The model under review builds one solid part; all positions refer to its coordinate system, in mm. A direction names the side the tool comes from. Coordinates: 2 decimals unless noted, no trailing zeros. Write each loop counter-clockwise with the first axis right and the second up, starting at its lowest first coordinate (ties: lowest second). Pieces come first, ordered by that corner, then holes. Notation, with made-up numbers: (14, 33) -> (72, 33) arc R14 cw to (72, 40) -> close; hole circle Ø9 at (8.5, -14.5). An arc over 180 degrees is marked (long way). Put each result on its own line as item: value. Start each with the question number.
from build123d import *

# Parameters (mm, degrees)
SKETCH_R          = 8.35
SKETCH_R_2        = 7.1
PAD_DEPTH         = 4
SKETCH001_W       = 35.5
SKETCH001_H       = 35.5
SKETCH001_R       = 6.6
PAD001_DEPTH      = 2
SKETCH002_W       = 4
SKETCH002_H       = 2
POCKET_DEPTH      = 25
POCKET_DEPTH_BACK = 25
FILLET002_R       = 0.5
SKETCH010_R       = 7.1
POCKET002_DEPTH   = 1


with BuildPart() as part:
    # Sketch → Pad (new body)
    with BuildSketch(Plane.XZ):
        Circle(SKETCH_R)
        Circle(SKETCH_R_2, mode=Mode.SUBTRACT)
    extrude(amount=PAD_DEPTH)

    # Sketch001 → Pad001 (join)
    with BuildSketch(Plane.XZ):
        with Locations((1.775, 0)):
            Rectangle(SKETCH001_W, SKETCH001_H)
        Circle(SKETCH001_R, mode=Mode.SUBTRACT)
    extrude(amount=-PAD001_DEPTH)

    # Sketch002 (on DatumPlane) → Pocket (cut, two sides)
    with BuildSketch(Plane.YZ) as pocket_sk:
        with Locations((-2, 0)):
            Rectangle(SKETCH002_W, SKETCH002_H)
    extrude(amount=-POCKET_DEPTH, mode=Mode.SUBTRACT)
    extrude(pocket_sk.sketch, amount=POCKET_DEPTH_BACK, mode=Mode.SUBTRACT)

    # Fillet002
    fillet002_edges = [part.edges().sort_by_distance(p)[0] for p in [
        (-15.975, 1, -17.75),
        (-15.975, 1, 17.75),
    ]]
    fillet(fillet002_edges, radius=FILLET002_R)

    # Sketch010 → Pocket002 (cut)
    with BuildSketch(Plane.XZ):
        Circle(SKETCH010_R)
    extrude(amount=-POCKET002_DEPTH, mode=Mode.SUBTRACT)


with BuildPart() as part_1:
    # Body placement: moved
    add(part.part.moved(Location((-2.5, -3, 0))))


solid = part_1.part
1. Tool access review of faces 1 (the cylindrical face through (4.272, -4.535, 2.133)), 2 (the flat face through (5, -5, 1)), 3 (the cylindrical face through (-2.67, -4.97, -8.35)): name each direction out of +Z, -Z, +X, -X, +Y, -Y from which nothing blocks a thin tool from reaching the whole face with its end or side.
2. Consider section D-D on z = -11. State the section outline as (x, y) points (3 decimals), then the cut area to 3 significant figures.
3. Consider section A-A on z = 0. State the section outline as (x, y) points (3 decimals), then the cut area to 3 significant figures.
4. Consider section B-B on x = -2.5. State the section outline as (y, z) points, then the cut area to 3 significant figures.
5. Wall thickness on line 1 (Z direction, x = -2.5, y = -4.5); line 2 (Z direction, x = -2.5, y = -1.5); line 3 (Y direction, x = -15, z = 12.5): over which ranges is each line inside the solid? List them lowest first. Write a range as from..to.
6. Insertion check: P1, Ø1.4, axis at x = 5.5, y = -6, coming from the -Z side; P2, Ø12, axis at x = -2.5, z = 0, coming from the -Y side; P3, Ø1, axis at x = 5.5, y = -4, coming from the +Z side; P4, Ø0.6, axis at x = -10.5, y = -5, coming from the +Z side. Each pin has a flat end and moves straight along its axis. Give the tip position at first contact, or say it passes through.
7. Consider section C-C on y = -4.8. State the section outline as (x, z) points, then the cut area to 3 significant figures.
Output values:
1. face 1: -Y
1. face 2: +X, -X, -Y
1. face 3: -Z, -Y
2. outline: (-18.475, -3) -> (17.025, -3) -> (17.025, -1) -> (-18.475, -1) -> close
2. area: 71.0 mm^2
3. outline: (-18.475, -3) -> (-9.6, -3) -> (-9.6, -2) -> (-9.1, -2) -> (-9.1, -1) -> (-18.475, -1) -> close; (4.1, -2) -> (4.6, -2) -> (4.6, -3) -> (17.025, -3) -> (17.025, -1) -> (4.1, -1) -> close
3. area: 43.6 mm^2
4. outline: (-7, -8.35) -> (-3, -8.35) -> (-3, -17.75) -> (-1, -17.75) -> (-1, -6.6) -> (-2, -6.6) -> (-2, -7.1) -> (-7, -7.1) -> close; (-7, 7.1) -> (-2, 7.1) -> (-2, 6.6) -> (-1, 6.6) -> (-1, 17.75) -> (-3, 17.75) -> (-3, 8.35) -> (-7, 8.35) -> close
4. area: 53.6 mm^2
5. line 1: z = -8.35..-7.1, 7.1..8.35
5. line 2: z = -17.75..-6.6, 6.6..17.75
5. line 3: y = -3..-1
6. P1: stops at z = -4.05
6. P2: passes through
6. P3: stops at z = 3.67
6. P4: stops at z = 3.23
7. outline: (-10.79, -1) arc R8.35 ccw to (5.79, -1) -> (4.53, -1) arc R7.1 cw to (-9.53, -1) -> close; (-10.79, 1) -> (-9.53, 1) arc R7.1 cw to (4.53, 1) -> (5.79, 1) arc R8.35 ccw to start
7. area: 55.7 mm^2
